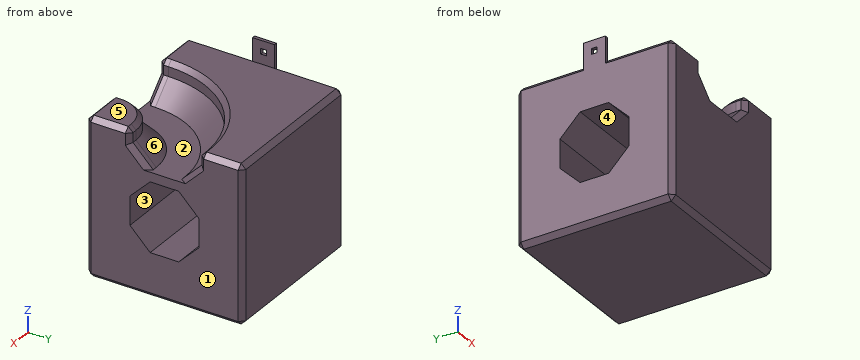
from build123d import *

# Parameters (mm, degrees)
SKETCH1_W                = 50
SKETCH1_H                = 50
BOSS_EXTRUDE1_DEPTH      = 50
CUT_EXTRUDE1_DEPTH       = 87.602540378
CHAMFER3_SIZE            = 1.5
BOSS_EXTRUDE2_DEPTH      = 7
BOSS_EXTRUDE2_DEPTH_BACK = 10
SKETCH5_W                = 1
SKETCH5_H                = 7
SKETCH6_W                = 1.8
SKETCH6_H                = 1.8
CUT_EXTRUDE2_DEPTH       = 7


with BuildPart() as part:
    # Sketch1 → Boss-Extrude1 (new body)
    with BuildSketch(Plane.XY):
        with Locations((25, 25)):
            Rectangle(SKETCH1_W, SKETCH1_H)
    extrude(amount=BOSS_EXTRUDE1_DEPTH)

    # Sketch2 → Cut-Extrude1 (cut, through all)
    with BuildSketch(Plane.ZY):
        Polygon((36, 29.556349186), (29.556349186, 36), (20.443650814, 36), (14, 29.556349186), (14, 20.443650814), (20.443650814, 14), (29.556349186, 14), (36, 20.443650814), align=None)
    extrude(amount=-CUT_EXTRUDE1_DEPTH, mode=Mode.SUBTRACT)

    # Cut-Sweep1: sweep along a path in Sketch4
    with BuildLine(Plane.XY.offset(50)) as cut_sweep1_path:
        Line((25, 0), (25, 3))
        ThreePointArc((25, 3), (31.443650814, 18.556349186), (47, 25))
        Line((47, 25), (50, 25))
    # Sketch3 → Cut-Sweep1 (sweep, cut)
    with BuildSketch(Plane.XZ):
        Polygon((29.556349186, 39), (36, 45.443650814), (36, 54.556349186), (29.556349186, 61), (20.443650814, 61), (14, 54.556349186), (14, 45.443650814), (20.443650814, 39), align=None)
    sweep(path=cut_sweep1_path.line, mode=Mode.SUBTRACT)

    # Chamfer3
    chamfer3_edges = [part.edges().sort_by_distance(p)[0] for p in [
        (50, 7, 50),
        (25, 50, 50),
        (43, 0, 50),
        (50, 43, 50),
        (36, 1.5, 50),
        (39.221825407, 10.778174593, 50),
        (48.5, 14, 50),
        (14, 1.5, 50),
        (23.665476221, 26.334523779, 50),
        (48.5, 36, 50),
        (50, 36, 47.721825407),
        (50, 14, 47.721825407),
        (36, 0, 47.721825407),
        (14, 0, 47.721825407),
        (17.221825407, 0, 42.221825407),
        (32.778174593, 0, 42.221825407),
        (50, 32.778174593, 42.221825407),
        (50, 17.221825407, 42.221825407),
        (0, 25, 50),
        (25, 50, 0),
        (50, 25, 0),
        (25, 0, 0),
        (0, 25, 0),
        (7, 0, 50),
        (0, 50, 25),
        (50, 50, 25),
        (50, 0, 25),
        (0, 0, 25),
    ]]
    chamfer(chamfer3_edges, length=CHAMFER3_SIZE)

    # Sketch5 → Boss-Extrude2 (add, two sides: drawn at the far end of the back side and taken through both)
    with BuildSketch(Plane.XY.offset(50).offset(-BOSS_EXTRUDE2_DEPTH_BACK)):
        with Locations((0.5, 25)):
            Rectangle(SKETCH5_W, SKETCH5_H)
    extrude(amount=BOSS_EXTRUDE2_DEPTH + BOSS_EXTRUDE2_DEPTH_BACK)

    # Sketch6 → Cut-Extrude2 (cut)
    with BuildSketch(Plane(origin=(1, 0, 0), x_dir=(0, 0, -1), z_dir=(1, 0, 0))):
        with Locations((-53.6, 25)):
            Rectangle(SKETCH6_W, SKETCH6_H)
    extrude(amount=-CUT_EXTRUDE2_DEPTH, mode=Mode.SUBTRACT)


solid = part.part
Verification items for the finished model (mm, model axes). Face numbers are marked on the shaded views. A direction names the side the tool comes from. Round coordinates to 2 decimals unless told otherwise and drop trailing zeros. Order: outer loops, then holes, each group sorted by start corner. A loop starts at its lowest first (then second) coordinate and runs counter-clockwise, first axis right, second up. Notation, with made-up numbers: (70.5, 49) -> (97.5, 49) arc R7 ccw to (97.5, 53) -> close; hole circle Ø2 at (36, 3.5). An arc over 180 degrees is marked (long way). Put each result on its own line as item: value.
1) Mould release check, pull along X, two halves, no side actions. Record for the marked faces 1, 2 and 3: +X half, -X half, draft (parallel to the pull), parting line (faces both ways), or undercut.
Final values:
face 1: +X half
face 2: undercut
face 3: draft
2) Section check B-B (y = 45). Record the cut outline in (x, z), then the cut area to 3 significant figures.
Final values:
outline: (0, 1.5) -> (1.5, 0) -> (48.5, 0) -> (50, 1.5) -> (50, 48.5) -> (48.5, 50) -> (1.5, 50) -> (0, 48.5) -> close
area: 2,500 mm^2
3) Section check D-D (z = 19). Record the cut outline in (x, y), then the cut area to 3 significant figures.
Final values:
outline: (0, 1.5) -> (1.5, 0) -> (48.5, 0) -> (50, 1.5) -> (50, 15.44) -> (0, 15.44) -> close; (0, 34.56) -> (50, 34.56) -> (50, 48.5) -> (48.5, 50) -> (1.5, 50) -> (0, 48.5) -> close
area: 1,540 mm^2
4) Section check A-A (z = 53.5). Record the cut outline in (x, y).
Final values:
outline: (0, 21.5) -> (1, 21.5) -> (1, 24.1) -> (0, 24.1) -> close; (0, 25.9) -> (1, 25.9) -> (1, 28.5) -> (0, 28.5) -> close
5) Section check C-C (z = 41). Record the cut outline in (x, y).
Final values:
outline: (0, 1.5) -> (1.5, 0) -> (16.32, 0) -> (18.44, 1.5) -> (18.44, 3) arc R28.56 cw to (47, 31.56) -> (48.5, 31.56) -> (50, 33.68) -> (50, 48.5) -> (48.5, 50) -> (1.5, 50) -> (0, 48.5) -> close; (31.56, 1.5) -> (33.68, 0) -> (48.5, 0) -> (50, 1.5) -> (50, 16.32) -> (48.5, 18.44) -> (47, 18.44) arc R15.44 ccw to (31.56, 3) -> close
6) Material ranges on line 1 (Y direction, x = 48, z = 46); line 2 (Z direction, x = 41.5, y = 22.5); line 3 (Z direction, x = 17, y = 38.5), recorded low to high.
Final values:
line 1: y = 0 to 14, 36 to 50
line 2: z = 0 to 14, 36 to 39
line 3: z = 0 to 50
7) Depth check by flat-ended pin: pin 1 (1.1 mm diameter, centred on x = 0.5, z = 53, fed in from +Y); pin 2 (16 mm diameter, centred on x = 40.5, y = 23, fed in from +Z); pin 3 (12 mm diameter, centred on x = 45, y = 9, fed in from +Z). Enter the tip coordinate at first touch or a pass-through.
Final values:
pin 1: stops at y = 28.5
pin 2: stops at z = 43.41
pin 3: stops at z = 50
8) Set-up check for the marked faces 4, 5 and 6: record each of +Z, -Z, +X, -X, +Y, -Y from which the full face is reachable in a straight line by a thin tool's end or side.
Final values:
face 4: +X, -X
face 5: +Z, +X, -X, +Y, -Y
face 6: +Z
